Could you check a few things on this model? Use its own coordinates, in mm. A direction names the side the tool comes from. Give positions to 0.01 mm unless a question says otherwise; leave off trailing zeros. Loops run counter-clockwise (first coordinate to the right, second up) from the corner with the lowest first, then second, coordinate; pieces in that order, holes last. Notation, with made-up numbers: M -6,16.25 L 12,16.25 A24 ccw 12,55.25 Z; hole C 14,43.5 d8. An arc over 180 degrees is marked long. Return JSON: item names as keys, results as strings. Group by question number.
1. If we section it at C-C (y = -19): Write out the boundary of the cut face in (x, z).
2. For pin 1 (4 mm diameter, centred on x = -71, y = 23.5, fed in from -Z); pin 2 (1 mm diameter, centred on y = -0.5, z = 30.5, fed in from -X); pin 3 (7.5 mm diameter, centred on y = 5.5, z = 34, fed in from -X); pin 4 (1 mm diameter, centred on y = 1.5, z = 15.5, fed in from +X), each with a flat end and sliding along its axis, tell me the tip position at first contact or that it passes through.
3. Please list where these lines run through material, in increasing order: line 1 (X direction, y = 0, z = 2.35); line 2 (X direction, y = 14.5, z = 2).
4. For faces 1 (the flat face through (-0.25, 64.4, 2.7)), 2 (the flat face through (-64.95, 0, 26)), 3 (the flat face through (-21, 21, 0)), which set-ups out of +Z, -Z, +X, -X, +Y, -Y let a thin tool reach every point of the face, with its end or its side?
5. If we section it at D-D (y = 72.5): Write out the boundary of the cut face in (x, z).
6. If we mould it in two halves opening along Y, with no side actions, what happens to faces 4 (the cylindrical face through (-65.597, 60.15, 1.479)), 5 (the flat face through (-21, 21, 3)), 6 (the flat face through (-14, -87, 3.2))? For each: +Y half, -Y half, draft (parallel to the pull), parting line (faces both ways), or undercut.
7. If we section it at A-A (z = 33): Write out the boundary of the cut face in (x, y).
8. If we section it at B-B (z = 5.5): Write out the boundary of the cut face in (x, y).
```python
from build123d import *

# Parameters (mm, degrees)
F0_R      = 89
F0_R_2    = 28.6
F1_DEPTH  = 3
F3_DEPTH  = 47
F6_DEPTH  = 9
F7_R      = 0.5
F9_DEPTH  = 0.2
F11_DEPTH = 9.5


with BuildPart() as f1:
    # F0 (on Top) → F1 (new body)
    with BuildSketch(Plane.XY):
        Circle(F0_R)
        Circle(F0_R_2, mode=Mode.SUBTRACT)
    extrude(amount=F1_DEPTH)

    # F2 (on face) → F3 (join)
    with BuildSketch(Plane.XY.offset(3)):
        Polygon((-64.95, 7.65), (-67.05, 7.65), (-67.05, 0.65), (-69.05, 0.65), (-69.05, -0.65), (-67.05, -0.65), (-67.05, -7.65), (-64.95, -7.65), align=None)
    extrude(amount=F3_DEPTH)

    # F4: F1 across plane


with BuildPart() as f1_1:
    add(f1.part)
    add(f1.part.mirror(Plane.YZ))

    # F5 (on face) → F6 (join)
    with BuildSketch(Plane.XY.offset(3)):
        with BuildLine():
            Line((-0.25, 55), (-0.25, 56.782554))
            ThreePointArc((-0.25, 56.782554), (0, 53.2), (0.25, 56.782554))
            Line((0.25, 56.782554), (0.25, 55))
            ThreePointArc((0.25, 55), (0, 54.75), (-0.25, 55))
        make_face()
    extrude(amount=F6_DEPTH)

    # F7
    f7_edges = [f1_1.edges().sort_by_distance(p)[0] for p in [
        (0, 53.2, 12),
    ]]
    fillet(f7_edges, radius=F7_R)

    # F8 (on face) → F9 (join)
    with BuildSketch(Plane.XY.offset(3)):
        with BuildLine():
            Line((87.556824, 2.75), (88.757408, 2.75))
            ThreePointArc((88.757408, 2.75), (0, 88.8), (-88.757408, 2.75))
            Line((-88.757408, 2.75), (-87.556824, 2.75))
            ThreePointArc((-87.556824, 2.75), (0, 87.6), (87.556824, 2.75))
        make_face()
        with BuildLine():
            Line((88.757408, -2.75), (87.556824, -2.75))
            ThreePointArc((87.556824, -2.75), (0, -87.6), (-87.556824, -2.75))
            Line((-87.556824, -2.75), (-88.757408, -2.75))
            ThreePointArc((-88.757408, -2.75), (0, -88.8), (88.757408, -2.75))
        make_face()
    extrude(amount=F9_DEPTH)

    # F10 (on face) → F11 (cut)
    with BuildSketch(Plane.XY.offset(12)):
        with BuildLine():
            Line((0.25, 55), (0.25, 56.275735))
            Line((0.25, 56.275735), (0.25, 92))
            Line((0.25, 92), (-0.25, 92))
            Line((-0.25, 92), (-0.25, 56.275735))
            Line((-0.25, 56.275735), (-0.25, 55))
            ThreePointArc((-0.25, 55), (0, 54.75), (0.25, 55))
        make_face()
    extrude(amount=-F11_DEPTH, mode=Mode.SUBTRACT)


solid = f1_1.part
```
Answer:
{
 "1": {"outline": "M -86.95,0 L -21.38,0 L -21.38,3 L -85.51,3 L -85.51,3.2 L -86.74,3.2 L -86.74,3 L -86.95,3 Z; M 21.38,0 L 86.95,0 L 86.95,3 L 86.74,3 L 86.74,3.2 L 85.51,3.2 L 85.51,3 L 21.38,3 Z"},
 "2": {"pin 1": "stops at z = 0", "pin 2": "stops at x = -69.05", "pin 3": "stops at x = -67.05", "pin 4": "stops at x = 67.05"},
 "3": {"line 1": "x = -89 to -28.6, 28.6 to 89", "line 2": "x = -87.81 to -24.65, 24.65 to 87.81"},
 "4": {"face 1": "+Z, +Y", "face 2": "+Z, +Y, -Y", "face 3": "-Z, +X, -X, +Y, -Y"},
 "5": {"outline": "M -51.62,0 L 51.62,0 L 51.62,3 L 51.28,3 L 51.28,3.2 L 49.17,3.2 L 49.17,3 L 0.25,3 L 0.25,2.5 L -0.25,2.5 L -0.25,3 L -49.17,3 L -49.17,3.2 L -51.28,3.2 L -51.28,3 L -51.62,3 Z"},
 "6": {"face 4": "parting line", "face 5": "undercut", "face 6": "draft"},
 "7": {"outline": "M -69.05,-0.65 L -67.05,-0.65 L -67.05,-7.65 L -64.95,-7.65 L -64.95,7.65 L -67.05,7.65 L -67.05,0.65 L -69.05,0.65 Z; M 64.95,-7.65 L 67.05,-7.65 L 67.05,-0.65 L 69.05,-0.65 L 69.05,0.65 L 67.05,0.65 L 67.05,7.65 L 64.95,7.65 Z"},
 "8": {"outline": "M -69.05,-0.65 L -67.05,-0.65 L -67.05,-7.65 L -64.95,-7.65 L -64.95,7.65 L -67.05,7.65 L -67.05,0.65 L -69.05,0.65 Z; M -0.25,55 L -0.25,56.78 A1.8 ccw long 0.25,56.78 L 0.25,55 A0.25 cw Z; M 64.95,-7.65 L 67.05,-7.65 L 67.05,-0.65 L 69.05,-0.65 L 69.05,0.65 L 67.05,0.65 L 67.05,7.65 L 64.95,7.65 Z"}
}
